Input: part model. Units: mm. Frame: model coordinates. Coordinates: 2 decimals unless noted, no trailing zeros. Write each loop counter-clockwise with the first axis right and the second up, starting at its lowest first coordinate (ties: lowest second). Pieces come first, ordered by that corner, then holes.
1) Section query B-B (x = 0.5). Output: boundary loops of the cut face in (y, z), then the cut area to 3 significant figures.
2) Section query C-C (x = 10). Output: boundary loops of the cut face in (y, z), then the cut area to 3 significant figures.
3) Pin query (flat end, axial travel): pin 1 Ø2 at (x, y) = (23.21, 0.04) entering from -Z. Return the tip coordinate at first contact, or that it passes through.
4) Line query: L1, parallel to X at y = 16, z = 0.45; L2, parallel to Y at x = 23.5, z = 1.35; L3, parallel to Y at x = -6, z = 0.95. Output: solid intervals per line, ascending.
5) Section query A-A (z = 1.6). State how many separate pieces and enclosed holes the cut face has, then the cut area to 3 significant figures.
from build123d import *

# Parameters (mm, degrees)
SKETCH_1_R      = 1.25
SKETCH_1_R_2    = 1
EXTRUDE_1_DEPTH = 2


with BuildPart() as part:
    # 草圖1 → 填料-伸長1 (new body)
    with BuildSketch(Plane.XY):
        with BuildLine():
            Line((25.714690816, 4.04468624), (25.714690816, -0.95531376))
            Line((25.714690816, -0.95531376), (25.714690816, -12.45531376))
            ThreePointArc((25.714690816, -12.45531376), (25.421797597, -13.162420542), (24.714690816, -13.45531376))
            Line((24.714690816, -13.45531376), (-14.285309184, -13.45531376))
            ThreePointArc((-14.285309184, -13.45531376), (-14.992415965, -13.162420542), (-15.285309184, -12.45531376))
            Line((-15.285309184, -12.45531376), (-15.285309184, 3.54468624))
            Line((-15.285309184, 3.54468624), (-15.285309184, 23.54468624))
            Line((-15.285309184, 23.54468624), (-15.285309184, 39.54468624))
            ThreePointArc((-15.285309184, 39.54468624), (-14.992415965, 40.251793021), (-14.285309184, 40.54468624))
            Line((-14.285309184, 40.54468624), (24.714690816, 40.54468624))
            ThreePointArc((24.714690816, 40.54468624), (25.421797597, 40.251793021), (25.714690816, 39.54468624))
            Line((25.714690816, 39.54468624), (25.714690816, 28.54468624))
            Line((25.714690816, 28.54468624), (25.714690816, 23.04468624))
            ThreePointArc((25.714690816, 23.04468624), (25.421797597, 22.337579458), (24.714690816, 22.04468624))
            Line((24.714690816, 22.04468624), (20.714690816, 22.04468624))
            ThreePointArc((20.714690816, 22.04468624), (20.007584035, 21.751793021), (19.714690816, 21.04468624))
            Line((19.714690816, 21.04468624), (19.714690816, 6.04468624))
            ThreePointArc((19.714690816, 6.04468624), (20.007584035, 5.337579458), (20.714690816, 5.04468624))
            Line((20.714690816, 5.04468624), (24.714690816, 5.04468624))
            ThreePointArc((24.714690816, 5.04468624), (25.421797597, 4.751793021), (25.714690816, 4.04468624))
        make_face()
        with Locations((-6.785309184, 27.04468624)):
            Circle(SKETCH_1_R, mode=Mode.SUBTRACT)
        with Locations((23.214690816, 27.04468624)):
            Circle(SKETCH_1_R, mode=Mode.SUBTRACT)
        with Locations((-6.785309184, 0.04468624)):
            Circle(SKETCH_1_R, mode=Mode.SUBTRACT)
        with Locations((23.214690816, 0.04468624)):
            Circle(SKETCH_1_R, mode=Mode.SUBTRACT)
        with Locations((-12.785309184, 33.04468624)):
            Circle(SKETCH_1_R, mode=Mode.SUBTRACT)
        with Locations((23.214690816, 33.04468624)):
            Circle(SKETCH_1_R, mode=Mode.SUBTRACT)
        with Locations(Location((23.214690816, -5.95531376, 0), (0, 0, 180))):
            Circle(SKETCH_1_R, mode=Mode.SUBTRACT)
        with Locations(Location((-12.785309184, -5.95531376, 0), (0, 0, 180))):
            Circle(SKETCH_1_R, mode=Mode.SUBTRACT)
        with Locations((-13.285309184, 19.54468624)):
            Circle(SKETCH_1_R_2, mode=Mode.SUBTRACT)
        with Locations((-13.285309184, 7.54468624)):
            Circle(SKETCH_1_R_2, mode=Mode.SUBTRACT)
        with BuildLine():
            Line((3.214690816, 22.04468624), (8.214690816, 22.04468624))
            ThreePointArc((8.214690816, 22.04468624), (11.750224722, 20.580220146), (13.214690816, 17.04468624))
            Line((13.214690816, 17.04468624), (13.214690816, 10.04468624))
            ThreePointArc((13.214690816, 10.04468624), (11.750224722, 6.509152334), (8.214690816, 5.04468624))
            Line((8.214690816, 5.04468624), (3.214690816, 5.04468624))
            ThreePointArc((3.214690816, 5.04468624), (-0.32084309, 6.509152334), (-1.785309184, 10.04468624))
            Line((-1.785309184, 10.04468624), (-1.785309184, 17.04468624))
            ThreePointArc((-1.785309184, 17.04468624), (-0.32084309, 20.580220146), (3.214690816, 22.04468624))
        make_face(mode=Mode.SUBTRACT)
    extrude(amount=EXTRUDE_1_DEPTH)


solid = part.part
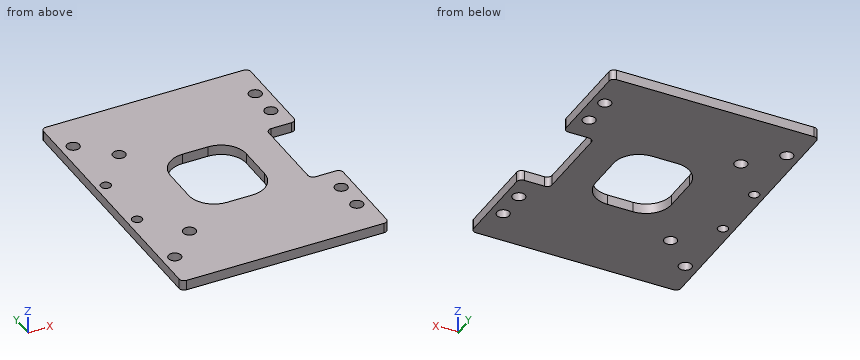
Answer:
1. outline: (-13.46, 0) - (5.85, 0) - (5.85, 2) - (-13.46, 2) - close; (21.24, 0) - (40.54, 0) - (40.54, 2) - (21.24, 2) - close
1. area: 77.2 mm2
2. outline: (-13.46, 0) - (5.37, 0) - (5.37, 2) - (-13.46, 2) - close; (21.72, 0) - (40.54, 0) - (40.54, 2) - (21.72, 2) - close
2. area: 75.3 mm2
3. pin 1: passes through
4. L1: x = -15.29 to -1.79, 13.21 to 19.71
4. L2: y = -13.46 to -7.17, -4.74 to -1.17, 1.26 to 5.04, 22.04 to 25.83, 28.26 to 31.83, 34.26 to 40.54
4. L3: y = -13.46 to -0.93, 1.02 to 26.07, 28.02 to 40.54
5. separate pieces: 1
5. enclosed holes: 11
5. area: 1,830 mm2
